Verification items for the finished model (mm, model axes). Coordinates: 2 decimals unless noted, no trailing zeros. Order: outer loops, then holes, each group sorted by start corner. A loop starts at its lowest first (then second) coordinate and runs counter-clockwise, first axis right, second up. Notation, with made-up numbers: M 18,40 L 35,40 A12 ccw 35,63 Z; hole C 6.25,78.5 d7. An arc over 180 degrees is marked long. Answer as a JSON object with one key per item and string values. Group by question number.
(1) Cross-section at A-A (y = 61). Enter the section's corners in (x, z) (3 decimals).
(2) Mould release check, pull along Y, two halves, no side actions. Record for faces 1 (the face through (-2.69, 81.46, 1.57)), 2 (the face through (11, 79, 0)), 3 (the face through (12.9, 81.24, 1.57)): released by +Y, released by -Y, zero draft, split by the parting line, or undercut.
(3) Gauge pin test, flat ends, axial feed: pin 1 Ø1.5 at (x, z) = (12.5, 1) entering from +Y; pin 2 Ø1.5 at (y, z) = (57, 1.5) entering from -X; pin 3 Ø1.5 at (x, z) = (4.5, 2) entering from -Y. Record the tip position at first contact, or that the pin passes through.
(4) Material ranges on line 1 (Y direction, x = 0, z = 1.15) (3 decimals); line 2 (X direction, y = 61.5, z = 2.5); line 3 (X direction, y = 69.5, z = 2.35), recorded low to high.
(5) Cross-section at B-B (x = -7.5). Enter the section's corners in (y, z) (3 decimals), plus the area to 3 significant figures.
(6) Cross-section at C-C (z = 2.2). Enter the section's corners in (x, y) (3 decimals).
from build123d import *

# Parameters (mm, degrees)
CYLINDER158_R     = 20.635
CYLINDER158_DEPTH = 41.275
CYLINDER157_R     = 24
CYLINDER157_DEPTH = 3.175


with BuildPart() as cylinder010:
    # Cylinder158 → Cylinder158 (new body)
    with BuildSketch(Plane.XY):
        Circle(CYLINDER158_R)
    extrude(amount=CYLINDER158_DEPTH)


with BuildPart() as cut020:
    # Cylinder157 → Cylinder157 (new body)
    with BuildSketch(Plane.XY):
        Circle(CYLINDER157_R)
    extrude(amount=CYLINDER157_DEPTH)

    # Cut020: cut Cylinder010
    add(cylinder010.part, mode=Mode.SUBTRACT)


with BuildPart() as cut020_1:
    # Cut020 placement: moved
    add(cut020.part.moved(Location((0, 61, 0))))


solid = cut020_1.part
Taken from the geometry:
{
 "1": {"outline": "M -24,0 L -20.635,0 L -20.635,3.175 L -24,3.175 Z; M 20.635,0 L 24,0 L 24,3.175 L 20.635,3.175 Z"},
 "2": {"face 1": "undercut", "face 2": "zero draft", "face 3": "split by the parting line"},
 "3": {"pin 1": "stops at y = 81.93", "pin 2": "stops at x = -23.78", "pin 3": "stops at y = 37.29"},
 "4": {"line 1": "y = 37 to 40.365, 81.635 to 85", "line 2": "x = -23.99 to -20.63, 20.63 to 23.99", "line 3": "x = -22.44 to -18.8, 18.8 to 22.44"},
 "5": {"outline": "M 38.202,0 L 41.776,0 L 41.776,3.175 L 38.202,3.175 Z; M 80.224,0 L 83.798,0 L 83.798,3.175 L 80.224,3.175 Z", "area": "22.7 mm²"},
 "6": {"outline": "C 0,61 d48; hole C 0,61 d41.27"}
}
